For this review, use the dimensioned drawing (mm, ordinates from the lowest corner) and the shaded views. A direction names the side the tool comes from. Round coordinates to 2 decimals unless told otherwise and drop trailing zeros. Loops run counter-clockwise (first coordinate to the right, second up) from the corner with the lowest first, then second, coordinate; pieces in that order, holes last. Notation, with made-up numbers: M 16,-34 L 27,-34 A16 cw 27,-22 Z; hole C 28,11 d9. An arc over 180 degrees is marked long. Answer as a JSON object with one key per item and string values. Group by question number.
Item 1: Insertion check: P1, Ø3, axis at y = 16, z = 3.5, coming from the -X side; P2, Ø2, axis at x = 38.5, y = 29, coming from the +Z side; P3, Ø4, axis at x = 40, y = 10, coming from the -Z side. Each pin has a flat end and moves straight along its axis. Give the tip position at first contact, or say it passes through.
Item 2: Consider section C-C (z = 4.5). Give the boundary of the cut face in (x, y), and give its area (3 significant figures).
Item 3: Consider section A-A (z = 15). Give the boundary of the cut face in (x, y), and give its area (3 significant figures).
Item 4: To check wall thickness, follow line 1 (X direction, y = 20, z = 6.75); line 2 (Y direction, x = 30, z = 13.75); line 3 (Y direction, x = 12.5, z = 18.5). State the ranges of each line that lie inside material, in increasing order.
Item 5: The part is to be moulded in two halves that separate along Y. For the marked faces 5, 6 and 7, say which applies: +Y half, -Y half, draft (parallel to the pull), parting line (faces both ways), or undercut.
Item 6: Tool access review of the marked faces 1, 2, 3 and 4: name each direction out of +Z, -Z, +X, -X, +Y, -Y from which nothing blocks a thin tool from reaching the whole face with its end or side.
Item 7: Consider section B-B (x = 52.5). Give the boundary of the cut face in (y, z).
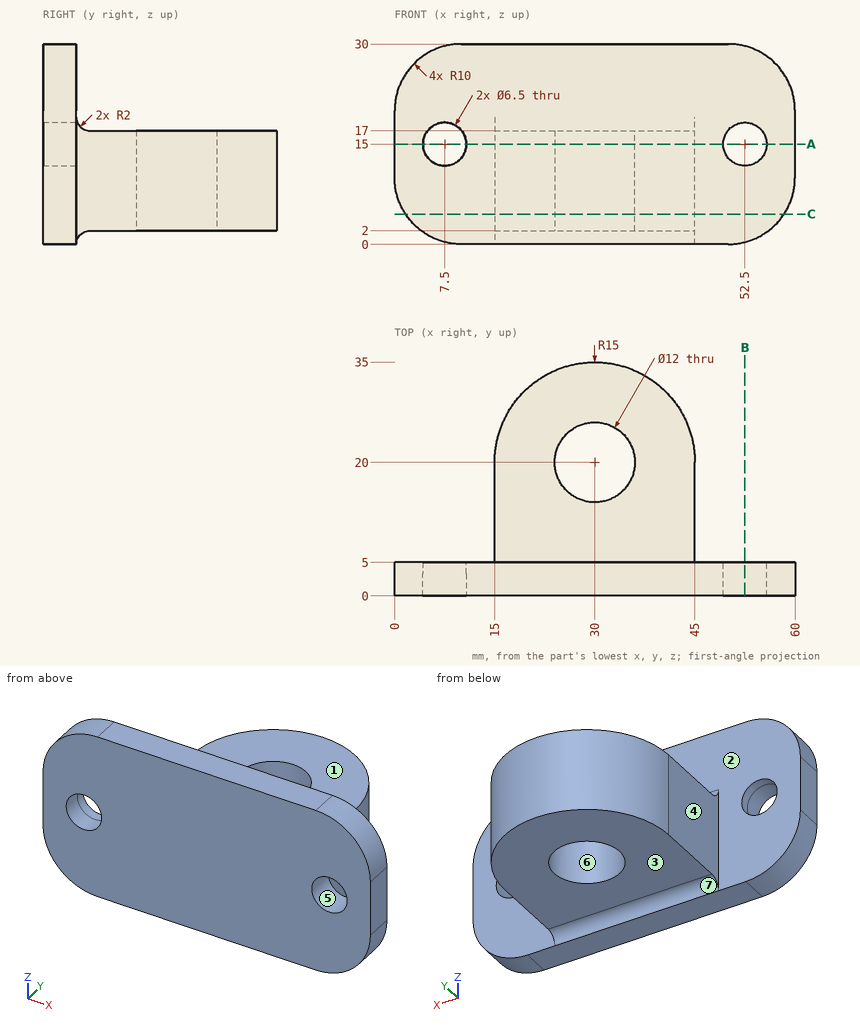
Geometry results:
{
 "1": {"P1": "stops at x = 15", "P2": "stops at z = 17", "P3": "stops at z = 2"},
 "2": {"outline": "M 1.65,0 L 58.35,0 L 58.35,5 L 45,5 L 45,20 A15 ccw 15,20 L 15,5 L 1.65,5 Z; hole C 30,20 d12", "area": "974 mm^2"},
 "3": {"outline": "M 0,0 L 4.25,0 L 4.25,5 L 0,5 Z; M 10.75,0 L 49.25,0 L 49.25,5 L 45,5 L 45,20 A15 ccw 15,20 L 15,5 L 10.75,5 Z; M 55.75,0 L 60,0 L 60,5 L 55.75,5 Z; hole C 30,20 d12", "area": "925 mm^2"},
 "4": {"line 1": "x = 15 to 24, 36 to 45", "line 2": "y = 0 to 14, 26 to 35", "line 3": "y = 0 to 5"},
 "5": {"face 5": "draft", "face 6": "undercut", "face 7": "+Y half"},
 "6": {"face 1": "+Z, +X, -X, +Y", "face 2": "+Z, +Y", "face 3": "-Z, +X, -X, +Y", "face 4": "+Z, -Z, -X, +Y"},
 "7": {"outline": "M 0,0.32 L 5,0.32 L 5,11.75 L 0,11.75 Z; M 0,18.25 L 5,18.25 L 5,29.68 L 0,29.68 Z"}
}
